```python
from build123d import *

# Parameters (mm, degrees)
SKETCH2_W           = 300
SKETCH2_H           = 430
BOSS_EXTRUDE1_DEPTH = 20
SKETCH3_R           = 15
CUT_EXTRUDE1_DEPTH  = 20
SKETCH4_R           = 34
CUT_EXTRUDE2_DEPTH  = 9.5
SKETCH5_R           = 7.5
BOSS_EXTRUDE2_DEPTH = 108.65
CUT_EXTRUDE4_START  = -25
SKETCH6_R           = 7.5
SKETCH6_R_2         = 5.5
CUT_EXTRUDE4_DEPTH  = 25
SKETCH7_W           = 20
SKETCH7_H           = 30
BOSS_EXTRUDE3_DEPTH = 78.65
SKETCH8_W           = 300
SKETCH8_H           = 218
BOSS_EXTRUDE4_DEPTH = 5
SKETCH12_R          = 2.5
CUT_EXTRUDE7_DEPTH  = 4
SKETCH13_W          = 36.95235035
SKETCH13_H          = 4.108205057
BOSS_EXTRUDE5_DEPTH = 78.6
SKETCH15_W          = 36.95235035
SKETCH15_H          = 4.108205057
BOSS_EXTRUDE6_DEPTH = 78.65
CUT_EXTRUDE8_DEPTH  = 474.234426579
SKETCH17_R          = 2.5
CUT_EXTRUDE9_DEPTH  = 474.234426579


with BuildPart() as part:
    # Sketch2 → Boss-Extrude1 (new body)
    with BuildSketch(Plane(origin=(0, 0, 0), x_dir=(1, 0, 0), z_dir=(0, 1, 0))):
        Rectangle(SKETCH2_W, SKETCH2_H)
    extrude(amount=BOSS_EXTRUDE1_DEPTH)

    # Sketch3 → Cut-Extrude1 (cut)
    with BuildSketch(Plane(origin=(0, 20, 0), x_dir=(1, 0, 0), z_dir=(0, 1, 0))):
        with Locations(Location((-75, 160, 0), (0, 0, 270))):
            Circle(SKETCH3_R)
        with Locations(Location((-75, -160, 0), (0, 0, 90))):
            Circle(SKETCH3_R)
    extrude(amount=-CUT_EXTRUDE1_DEPTH, mode=Mode.SUBTRACT)

    # Sketch4 → Cut-Extrude2 (cut)
    with BuildSketch(Plane(origin=(0, 20, 0), x_dir=(1, 0, 0), z_dir=(0, 1, 0))):
        with Locations(Location((-75, 160, 0), (0, 0, 270))):
            Circle(SKETCH4_R)
        with Locations(Location((-75, -160, 0), (0, 0, 90))):
            Circle(SKETCH4_R)
    extrude(amount=-CUT_EXTRUDE2_DEPTH, mode=Mode.SUBTRACT)

    # Sketch5 → Boss-Extrude2 (add)
    with BuildSketch(Plane(origin=(0, 20, 0), x_dir=(1, 0, 0), z_dir=(0, 1, 0))):
        with Locations(Location((81.635568617, 160, 0), (0, 0, 90))):
            Circle(SKETCH5_R)
        with Locations(Location((81.635568617, -160, 0), (0, 0, 90))):
            Circle(SKETCH5_R)
    extrude(amount=BOSS_EXTRUDE2_DEPTH)

    # Sketch6 → Cut-Extrude4 (cut)
    # profile 1 of 2: a face of its own
    with BuildSketch(Plane(origin=(0, 128.65, 0), x_dir=(1, 0, 0), z_dir=(0, 1, 0)).offset(CUT_EXTRUDE4_START)):
        with Locations(Location((81.635568617, -160, 0), (0, 0, 90))):
            Circle(SKETCH6_R)
        with Locations(Location((81.635568617, -160, 0), (0, 0, 270))):
            Circle(SKETCH6_R_2, mode=Mode.SUBTRACT)
    # profile 2 of 2: a face of its own
    with BuildSketch(Plane(origin=(0, 128.65, 0), x_dir=(1, 0, 0), z_dir=(0, 1, 0)).offset(CUT_EXTRUDE4_START)):
        with Locations(Location((81.635568617, 160, 0), (0, 0, 90))):
            Circle(SKETCH6_R)
        with Locations(Location((81.635568617, 160, 0), (0, 0, 90))):
            Circle(SKETCH6_R_2, mode=Mode.SUBTRACT)
    extrude(amount=CUT_EXTRUDE4_DEPTH, mode=Mode.SUBTRACT)

    # Sketch7 → Boss-Extrude3 (add)
    with BuildSketch(Plane(origin=(0, 20, 0), x_dir=(1, 0, 0), z_dir=(0, 1, 0))):
        with Locations((120, 0)):
            Rectangle(SKETCH7_W, SKETCH7_H)
        with Locations((-120, 0)):
            Rectangle(SKETCH7_W, SKETCH7_H)
    extrude(amount=BOSS_EXTRUDE3_DEPTH)

    # Sketch8 → Boss-Extrude4 (add)
    with BuildSketch(Plane(origin=(0, 98.65, 0), x_dir=(1, 0, 0), z_dir=(0, 1, 0))):
        Rectangle(SKETCH8_W, SKETCH8_H)
    extrude(amount=BOSS_EXTRUDE4_DEPTH)

    # Sketch12 → Cut-Extrude7 (cut)
    with BuildSketch(Plane.XZ.offset(-98.65)):
        with Locations(Location((144.5, 80.981198611, 0), (0, 0, 270))):
            Circle(SKETCH12_R)
        with Locations(Location((144.5, 36.981198611, 0), (0, 0, 270))):
            Circle(SKETCH12_R)
        with Locations(Location((144.5, -80.981198611, 0), (0, 0, 90))):
            Circle(SKETCH12_R)
        with Locations(Location((144.5, -36.981198611, 0), (0, 0, 90))):
            Circle(SKETCH12_R)
    extrude(amount=-CUT_EXTRUDE7_DEPTH, mode=Mode.SUBTRACT)

    # Sketch13 → Boss-Extrude5 (add)
    with BuildSketch(Plane(origin=(0, 20, 0), x_dir=(1, 0, 0), z_dir=(0, 1, 0))):
        with Locations((131.523824825, -212.945897472)):
            Rectangle(SKETCH13_W, SKETCH13_H)
    extrude(amount=BOSS_EXTRUDE5_DEPTH)

    # Sketch15 → Boss-Extrude6 (add)
    with BuildSketch(Plane(origin=(0, 20, 0), x_dir=(1, 0, 0), z_dir=(0, 1, 0))):
        with Locations((131.523824825, 212.945897472)):
            Rectangle(SKETCH15_W, SKETCH15_H)
    extrude(amount=BOSS_EXTRUDE6_DEPTH)

    # Sketch16 → Cut-Extrude8 (cut, through all)
    with BuildSketch(Plane.XY.offset(215)):
        Polygon((90.986671156, 0), (150, 26.663239915), (150, 0), align=None)
    extrude(amount=-CUT_EXTRUDE8_DEPTH, mode=Mode.SUBTRACT)

    # Sketch17 → Cut-Extrude9 (cut, through all)
    with BuildSketch(Plane.XY.offset(215)):
        with Locations((-50, 7)):
            Circle(SKETCH17_R)
    extrude(amount=-CUT_EXTRUDE9_DEPTH, mode=Mode.SUBTRACT)


solid = part.part
```
Check sheet for the modelled part. Datum: model origin and axes. Units: mm. A direction names the side the tool comes from. Round coordinates to 2 decimals unless told otherwise and drop trailing zeros. Order: outer loops, then holes, each group sorted by start corner. A loop starts at its lowest first (then second) coordinate and runs counter-clockwise, first axis right, second up. Notation, with made-up numbers: (14.5, -22) -> (72.5, -22) arc R31 ccw to (72.5, 5) -> close; hole circle Ø3 at (-28.5, 83). An arc over 180 degrees is marked (long way). One line per item, written item: value. Start each with the question number.
Q1. Cross-section at C-C (x = -75). Record the boundary of the cut face in (y, z).
Q2. Cross-section at B-B (x = 49.5). Record the boundary of the cut face in (y, z), and give its area (3 significant figures).
Q3. Set-up check for faces 5 (the face through (84.508, 61.239, -166.928)), 6 (the face through (-130, 59, 0)), 7 (the face through (130, 59, 0)): record each of +Z, -Z, +X, -X, +Y, -Y from which the full face is reachable in a straight line by a thin tool's end or side.
Q4. Cross-section at D-D (y = 31). Record the boundary of the cut face in (x, z).
Q5. Mould release check, pull along Y, two halves, no side actions. Record for faces 1 (the face through (-90, 10.5, -153)), 2 (the face through (113.52, 10.18, 3.01)), 3 (the face through (-9, 20, -3)), 4 (the face through (22, 13, -215)): pulls with the +Y half, pulls with the -Y half, needs draft (parallel to the pull), parting line crosses it, or undercut.
Q6. Thickness scan on line 1 (Z direction, x = 144, y = 101); line 2 (Z direction, x = 121.5, y = 67); line 3 (Y direction, x = 68, z = 31.5). Record the ranges inside material, lowest first.
Q7. Cross-section at A-A (z = -93). Record the boundary of the cut face in (x, y), and give its area (3 significant figures).
Q8. Gauge pin test, flat ends, axial feed: pin 1 Ø24 at (y, z) = (77, 4.5) entering from -X; pin 2 Ø4 at (x, z) = (144.5, -81) entering from -Y; pin 3 Ø4 at (x, y) = (5.5, 101.5) entering from +Z. Record the tip position at first contact, or that the pin passes through.
Completed:
1. outline: (0, -215) -> (20, -215) -> (20, -194) -> (10.5, -194) -> (10.5, -175) -> (0, -175) -> close; (0, -145) -> (10.5, -145) -> (10.5, -126) -> (20, -126) -> (20, 126) -> (10.5, 126) -> (10.5, 145) -> (0, 145) -> close; (0, 175) -> (10.5, 175) -> (10.5, 194) -> (20, 194) -> (20, 215) -> (0, 215) -> close; (98.65, -109) -> (103.65, -109) -> (103.65, 109) -> (98.65, 109) -> close
2. outline: (0, -215) -> (20, -215) -> (20, 215) -> (0, 215) -> close; (98.65, -109) -> (103.65, -109) -> (103.65, 109) -> (98.65, 109) -> close
2. area: 9,690 mm²
3. face 5: +Y
3. face 6: +Z, -Z, -X
3. face 7: +X
4. outline: (-130, -15) -> (-110, -15) -> (-110, 15) -> (-130, 15) -> close; circle Ø15 at (81.64, -160); circle Ø15 at (81.64, 160); (110, -15) -> (130, -15) -> (130, 15) -> (110, 15) -> close; (113.05, -215) -> (150, -215) -> (150, -210.89) -> (113.05, -210.89) -> close; (113.05, 210.89) -> (150, 210.89) -> (150, 215) -> (113.05, 215) -> close
5. face 1: pulls with the +Y half
5. face 2: pulls with the -Y half
5. face 3: undercut
5. face 4: needs draft
6. line 1: z = -109 to -83.43, -78.53 to -39.43, -34.53 to 34.53, 39.43 to 78.53, 83.43 to 109
6. line 2: z = -215 to -210.89, -15 to 15, 210.89 to 215
6. line 3: y = 0 to 20, 98.65 to 103.65
7. outline: (-150, 0) -> (90.99, 0) -> (135.25, 20) -> (-150, 20) -> close; (-150, 98.65) -> (150, 98.65) -> (150, 103.65) -> (-150, 103.65) -> close; hole circle Ø5 at (-50, 7)
7. area: 6,740 mm²
8. pin 1: stops at x = -130
8. pin 2: stops at y = 102.65
8. pin 3: stops at z = 109
